```python
from build123d import *

# Parameters (mm, degrees)
SKETCH1_R           = 1.5
BOSS_EXTRUDE1_DEPTH = 2


with BuildPart() as part:
    # Sketch1 → Boss-Extrude1 (new body)
    with BuildSketch(Plane.XY):
        with BuildLine():
            Line((5, 0), (9, 0))
            Line((9, 0), (9, 4))
            Line((9, 4), (13, 4))
            Line((13, 4), (13, 0))
            Line((13, 0), (17, 0))
            Line((17, 0), (17, 4))
            Line((17, 4), (19.021561934, 4))
            Line((19.021561934, 4), (19.021561934, 0))
            Line((19.021561934, 0), (38.059495851, 0))
            ThreePointArc((38.059495851, 0), (44.762590659, 5.991570372), (39.557599026, 13.322222296))
            Line((39.557599026, 13.322222296), (19.021561934, 17.999988357))
            Line((19.021561934, 17.999988357), (19.021561934, 13.999988357))
            Line((19.021561934, 13.999988357), (17, 13.999988357))
            Line((17, 13.999988357), (17, 17.999988357))
            Line((17, 17.999988357), (13, 17.999988357))
            Line((13, 17.999988357), (13, 13.999988357))
            Line((13, 13.999988357), (9, 13.999988357))
            Line((9, 13.999988357), (9, 17.999988357))
            Line((9, 17.999988357), (5, 17.999988357))
            Line((5, 17.999988357), (5, 13.999988357))
            Line((5, 13.999988357), (0, 13.999988357))
            Line((0, 13.999988357), (0, 4))
            Line((0, 4), (5, 4))
            Line((5, 4), (5, 0))
        make_face()
        with Locations((3.920490093, 9)):
            Circle(SKETCH1_R, mode=Mode.SUBTRACT)
        with Locations((38.059495851, 6.745343083)):
            Circle(SKETCH1_R, mode=Mode.SUBTRACT)
    extrude(amount=BOSS_EXTRUDE1_DEPTH)


solid = part.part
```
Check sheet for the modelled part. Datum: model origin and axes. Units: mm. A direction names the side the tool comes from. Coordinates: 2 decimals unless noted, no trailing zeros. Loops run counter-clockwise (first coordinate to the right, second up) from the corner with the lowest first, then second, coordinate; pieces in that order, holes last.
1) Sectioned sample at B-B (z = 1.4). Record the boundary of the cut face in (x, y), and give its area (3 significant figures).
2) Sectioned sample at A-A (y = 3). Record the boundary of the cut face in (x, z), and give its area (3 significant figures).
3) Release check for a two-part mould opening along X. For faces 1 (the face through (9, 2, 1)), 2 (the face through (44.746, 5.855, 0.986)), 3 (the face through (15, 18, 1)), 4 (the face through (17, 16, 1)) record: released by +X, released by -X, zero draft, split by the parting line, or undercut.
4) Gauge pin test, flat ends, axial feed: pin 1 (0.6 mm diameter, centred on x = 3.5, z = 0.5, fed in from -Y); pin 2 (1 mm diameter, centred on x = 40, z = 1, fed in from +Y); pin 3 (0.6 mm diameter, centred on y = 2, z = 1, fed in from -X); pin 4 (1.8 mm diameter, centred on x = 3.92, y = 9, fed in from +Z). Record the tip position at first contact, or that the pin passes through.
5) Sectioned sample at C-C (x = 4). Record the boundary of the cut face in (y, z).
6) Access from +Z, -Z, +X, -X, +Y, -Y to the whole of each face (thin tool, end or side, straight path). Record for faces 5 (the face through (18, 14, 1)), 6 (the face through (18, 4, 1)), 7 (the face through (3, 14, 1)), 8 (the face through (5, 2, 1)).
7) Sectioned sample at D-D (y = 6). Record the boundary of the cut face in (x, z).
8) Material ranges on probe 1 along X at (y, z) = (3.5, 0.45); probe 2 along X at (y, z) = (3, 1.65); probe 3 along Y at (x, z) = (4.5, 0.3), recorded low to high.
Check sheet entries:
1. outline: (0, 4) - (5, 4) - (5, 0) - (9, 0) - (9, 4) - (13, 4) - (13, 0) - (17, 0) - (17, 4) - (19.02, 4) - (19.02, 0) - (38.06, 0) arc R6.75 ccw to (39.56, 13.32) - (19.02, 18) - (19.02, 14) - (17, 14) - (17, 18) - (13, 18) - (13, 14) - (9, 14) - (9, 18) - (5, 18) - (5, 14) - (0, 14) - close; hole circle Ø3 at (3.92, 9); hole circle Ø3 at (38.06, 6.75)
1. area: 613 mm2
2. outline: (5, 0) - (9, 0) - (9, 2) - (5, 2) - close; (13, 0) - (17, 0) - (17, 2) - (13, 2) - close; (19.02, 0) - (43.67, 0) - (43.67, 2) - (19.02, 2) - close
2. area: 65.3 mm2
3. face 1: undercut
3. face 2: released by +X
3. face 3: zero draft
3. face 4: undercut
4. pin 1: stops at y = 4
4. pin 2: stops at y = 13.34
4. pin 3: stops at x = 5
4. pin 4: passes through
5. outline: (4, 0) - (7.5, 0) - (7.5, 2) - (4, 2) - close; (10.5, 0) - (14, 0) - (14, 2) - (10.5, 2) - close
6. face 5: +Z, -Z, +Y
6. face 6: +Z, -Z, -Y
6. face 7: +Z, -Z, -X, +Y
6. face 8: +Z, -Z, -X, -Y
7. outline: (0, 0) - (36.76, 0) - (36.76, 2) - (0, 2) - close; (39.36, 0) - (44.76, 0) - (44.76, 2) - (39.36, 2) - close
8. probe 1: x = 5 to 9, 13 to 17, 19.02 to 43.97
8. probe 2: x = 5 to 9, 13 to 17, 19.02 to 43.67
8. probe 3: y = 4 to 7.62, 10.38 to 14
